from build123d import *

# Parameters (mm, degrees)
F0_W     = 39.9214811623
F0_H     = 63.9728531241
F1_DEPTH = 25.4
F3_DEPTH = 62.738
F4_R     = 10.5479626422
F5_DEPTH = 43.18


with BuildPart() as f1:
    # F0 (on Right) → F1 (new body)
    with BuildSketch(Plane.YZ):
        with Locations((-19.9607405812, 31.9864265621)):
            Rectangle(F0_W, F0_H)
        Polygon((0, 63.9728531241), (0, 0), (37.7500206232, 0), align=None)
    extrude(amount=F1_DEPTH)

    # F2 (on Right) → F3 (join)
    with BuildSketch(Plane.YZ):
        Polygon((-39.7544465959, 63.8058185577), (-39.9214811623, 0), (25.3893956542, 0), (-9.0199168772, 63.8058185577), align=None)
    extrude(amount=-F3_DEPTH)

    # F4 (on face) → F5 (cut)
    with BuildSketch(Plane(origin=(0, 19.6691261726, 10.6072004872), x_dir=(-1, 0, 0), z_dir=(0, 0.8801695735, 0.4746593746))):
        with Locations((26.5113729984, 24.7412994504)):
            Circle(F4_R)
    extrude(amount=-F5_DEPTH, mode=Mode.SUBTRACT)


solid = f1.part
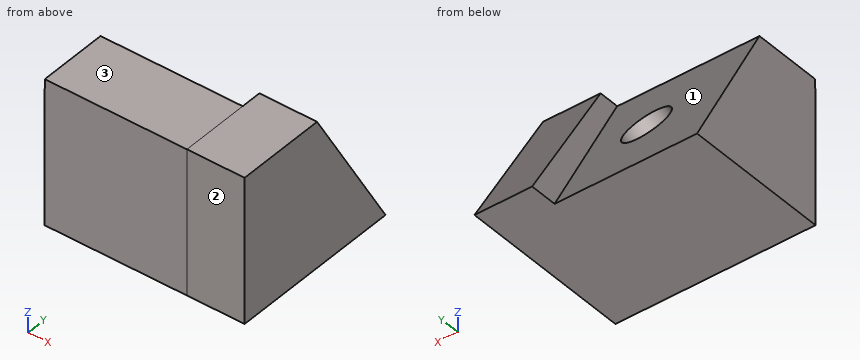
The model under review builds one solid part; all positions refer to its coordinate system, in mm. Face numbers are marked on the shaded views. A direction names the side the tool comes from. Round coordinates to 2 decimals unless told otherwise and drop trailing zeros. Loops run counter-clockwise (first coordinate to the right, second up) from the corner with the lowest first, then second, coordinate; pieces in that order, holes last. Notation, with made-up numbers: (-7, 38.5) -> (10, 38.5) arc R25 ccw to (10, 74.5) -> close; hole circle Ø7 at (23, 41). An arc over 180 degrees is marked (long way). Write item = value, one per line. Start each with the question number.
Item 1: For the marked faces 1, 2 and 3, list the 3-axis set-ups (+Z, -Z, +X, -X, +Y, -Y) from which the entire face can be reached by the end or side of a thin tool; tool diameter is ignored.
Item 2: Insertion check: pin 1 (9 mm diameter, centred on x = -40, y = -22.5, fed in from +Z); pin 2 (10 mm diameter, centred on y = 28, z = 17, fed in from -X); pin 3 (10 mm diameter, centred on x = -41, z = 55.5, fed in from +Y). Each pin has a flat end and moves straight along its axis. Give the tip position at first contact, or say it passes through.
Item 3: To check wall thickness, follow L1, parallel to X at y = 5.5, z = 25.5; L2, parallel to X at y = 9.5, z = 43; L3, parallel to Y at x = -34.5, z = 18. State the ranges of each line that lie inside material, in increasing order.
Item 4: Take a section at A-A on x = -24.5. Give the boundary of the cut face in (y, z), plus the area to 3 significant figures.
Item 5: Take a section at B-B on y = 16. Give the boundary of the cut face in (x, z), plus the area to 3 significant figures.
Item 6: Take a section at C-C on x = 12. Give the boundary of the cut face in (y, z).
Item 7: Take a section at D-D on x = -39.5. Give the boundary of the cut face in (y, z), plus the area to 3 significant figures.
Result:
q1.face_1 = +Z, -X, +Y
q1.face_2 = +Z, -Z, +X, -X, -Y
q1.face_3 = +Z, -X, +Y, -Y
q2.pin_1 = 63.81
q2.pin_2 = 0
q2.pin_3 = -1.84
q3.L1 = -62.74 to -35.85, -17.17 to 25.4
q3.L2 = 0 to 25.4
q3.L3 = -39.87 to -33.26, -4.24 to 15.68
q4.outline = (-39.92, 0) -> (25.39, 0) -> (12.84, 23.27) -> (-25.17, 2.77) -> (-35, 21) -> (3.01, 41.5) -> (-9.02, 63.81) -> (-39.75, 63.81) -> close
q4.area = 2,170 mm²
q5.outline = (-62.74, 0) -> (25.4, 0) -> (25.4, 36.86) -> (0, 36.86) -> (0, 17.41) -> (-62.74, 17.41) -> close
q5.area = 2,030 mm²
q6.outline = (-39.92, 0) -> (37.75, 0) -> (0, 63.97) -> (-39.92, 63.97) -> close
q7.outline = (-39.92, 0) -> (25.39, 0) -> (-9.02, 63.81) -> (-39.75, 63.81) -> close
q7.area = 3,060 mm²
